Geometry check sheet. Reference: the model listing, model coordinates, mm. Face numbers are marked on the shaded views. A direction names the side the tool comes from. Give positions to 0.01 mm unless a question says otherwise; leave off trailing zeros. Order: outer loops, then holes, each group sorted by start corner. A loop starts at its lowest first (then second) coordinate and runs counter-clockwise, first axis right, second up. Notation, with made-up numbers: M -24.5,81 L -3.5,81 A8 ccw -3.5,91 Z; hole C -10.5,83 d4. An arc over 180 degrees is marked long. Answer as CSV lines item,"result".
from build123d import *

# Parameters (mm, degrees)
SKETCH1_W           = 101.6
SKETCH1_H           = 50.8
SKETCH1_R           = 3.175
SKETCH1_R_2         = 1.27
SKETCH1_R_3         = 6.35
SKETCH1_W_2         = 43.18
SKETCH1_H_2         = 20.32
BOSS_EXTRUDE1_DEPTH = 9.525
SKETCH2_R           = 1.7272
CUT_EXTRUDE1_DEPTH  = 12.7


with BuildPart() as part:
    # Sketch1 → Boss-Extrude1 (new body)
    with BuildSketch(Plane.XY):
        with Locations((50.8, 25.4)):
            Rectangle(SKETCH1_W, SKETCH1_H)
        with Locations((95.25, 22.225)):
            Circle(SKETCH1_R, mode=Mode.SUBTRACT)
        with Locations((95.25, 9.525)):
            Circle(SKETCH1_R, mode=Mode.SUBTRACT)
        with Locations((3.048, 43.815)):
            Circle(SKETCH1_R_2, mode=Mode.SUBTRACT)
        with Locations((3.048, 31.115)):
            Circle(SKETCH1_R_2, mode=Mode.SUBTRACT)
        with Locations((52.832, 43.815)):
            Circle(SKETCH1_R_2, mode=Mode.SUBTRACT)
        with Locations((52.832, 31.115)):
            Circle(SKETCH1_R_2, mode=Mode.SUBTRACT)
        with Locations((70.435623446, 11.349127288)):
            Circle(SKETCH1_R_3, mode=Mode.SUBTRACT)
        with Locations((27.94, 37.465)):
            Rectangle(SKETCH1_W_2, SKETCH1_H_2, mode=Mode.SUBTRACT)
    extrude(amount=BOSS_EXTRUDE1_DEPTH)

    # Sketch2 → Cut-Extrude1 (cut)
    with BuildSketch(Plane.XZ):
        with Locations((60.2488, 4.7625)):
            Circle(SKETCH2_R)
        with Locations((79.2988, 4.7625)):
            Circle(SKETCH2_R)
    extrude(amount=-CUT_EXTRUDE1_DEPTH, mode=Mode.SUBTRACT)


solid = part.part
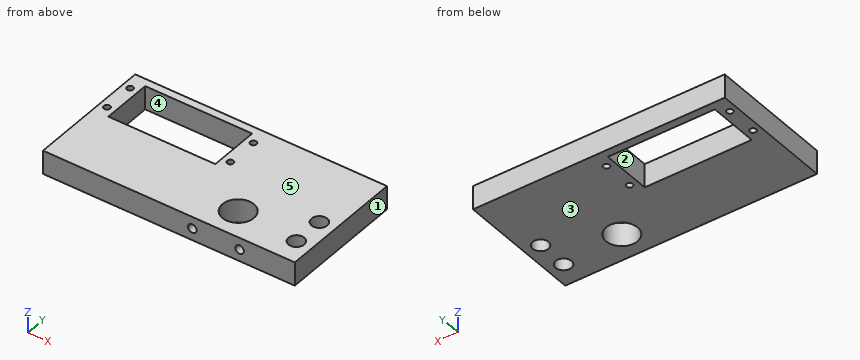
(1) Material ranges on line 1 (X direction, y = 44, z = 2.5); line 2 (Y direction, x = 95.25, z = 7); line 3 (X direction, y = 22, z = 5.75), recorded low to high.
The answers:
line 1,"x = 0 to 1.79, 4.3 to 6.35, 49.53 to 51.58, 54.09 to 101.6"
line 2,"y = 0 to 6.35, 12.7 to 19.05, 25.4 to 50.8"
line 3,"x = 0 to 92.08, 98.42 to 101.6"
(2) Section check B-B on y = 8. Enter the section's corners in (x, z) (1 decimal), then the cut area to 3 significant figures.
The answers:
outline,"M 0,0 L 65,0 L 65,9.5 L 0,9.5 Z; M 75.8,0 L 92.5,0 L 92.5,9.5 L 75.8,9.5 Z; M 98,0 L 101.6,0 L 101.6,9.5 L 98,9.5 Z; hole C 60.2,4.8 d3.5; hole C 79.3,4.8 d3.5"
area,"793 mm2"
(3) Section check D-D on x = 52.5. Enter the section's corners in (y, z) (3 decimals), then the cut area to 3 significant figures.
The answers:
outline,"M 0,0 L 29.889,0 L 29.889,9.525 L 0,9.525 Z; M 32.341,0 L 42.589,0 L 42.589,9.525 L 32.341,9.525 Z; M 45.041,0 L 50.8,0 L 50.8,9.525 L 45.041,9.525 Z"
area,"437 mm2"
(4) Section check C-C on z = 1.75. State how many separate pieces and enclosed holes the cut face has, then the cut area to 3 significant figures.
The answers:
separate pieces,"1"
enclosed holes,"8"
area,"4,070 mm2"
(5) Tool access check on the marked faces 4 and 5. Record the directions out of +Z, -Z, +X, -X, +Y, -Y that give a thin tool (end or side, any length) a straight path to the whole face; none if there is none.
The answers:
face 4,"+Z, -Z"
face 5,"+Z, +X, -X, +Y, -Y"
(6) Gauge pin test, flat end, axial feed: P1, Ø2, axis at x = 52.832, y = 31.115, coming from the -Z side. Record the tip position at first contact, or that the pin passes through.
The answers:
P1,"passes through"
(7) Draft check along X on the marked faces 1, 2 and 3. Enter one of: +X half, -X half, draft (parallel to the pull), parting line (faces both ways), or undercut.
The answers:
face 1,"+X half"
face 2,"undercut"
face 3,"draft"
(8) Section check A-A on x = 95.25. Enter the section's corners in (y, z) (3 decimals).
The answers:
outline,"M 0,0 L 6.35,0 L 6.35,9.525 L 0,9.525 Z; M 12.7,0 L 19.05,0 L 19.05,9.525 L 12.7,9.525 Z; M 25.4,0 L 50.8,0 L 50.8,9.525 L 25.4,9.525 Z"
